from build123d import *

# Parameters (mm, degrees)
SKETCH1_R           = 6
BOSS_EXTRUDE1_DEPTH = 50
SKETCH2_R           = 5.5
CUT_EXTRUDE1_DEPTH  = 50
FILLET1_R           = 1
FILLET2_R           = 1


with BuildPart() as part:
    # Sketch1 → Boss-Extrude1 (new body)
    with BuildSketch(Plane(origin=(0, 0, 0), x_dir=(1, 0, 0), z_dir=(0, 1, 0))):
        with Locations(Location((0, 0, 0), (0, 0, 270))):
            Circle(SKETCH1_R)
    extrude(amount=BOSS_EXTRUDE1_DEPTH)

    # Sketch2 → Cut-Extrude1 (cut)
    with BuildSketch(Plane(origin=(0, 50, 0), x_dir=(1, 0, 0), z_dir=(0, 1, 0))):
        with Locations(Location((0, 0, 0), (0, 0, 270))):
            Circle(SKETCH2_R)
    extrude(amount=-CUT_EXTRUDE1_DEPTH, mode=Mode.SUBTRACT)

    # Fillet1
    # the kernel refuses this fillet: 1 mm, written as the material it takes off along each edge
    with BuildSketch(Plane(origin=(0, 50, 0), x_dir=(0, 0, 1), z_dir=(-1, 0, 0))) as fillet1_piece_1:
        with BuildLine():
            CenterArc((5, -0.866025404), FILLET1_R, 0, 60)
            Line((5.5, 0), (5.51, 0.017320508))
            ThreePointArc((5.51, 0.017320508), (5.75, 0.02), (6, 0.02))
            Line((6, 0.02), (6.02, 0))
            Line((6.02, 0), (6.02, -0.866025404))
            Line((6.02, -0.866025404), (6, -0.866025404))
        make_face()
    revolve(axis=Axis((0, 50, 0), (0, 1, 0)), mode=Mode.SUBTRACT)

    # Fillet2
    # the kernel refuses this fillet: 1 mm, written as the material it takes off along each edge
    with BuildSketch(Plane(origin=(0, 0, 0), x_dir=(0, 0, 1), z_dir=(-1, 0, 0))) as fillet2_piece_1:
        with BuildLine():
            CenterArc((5, 0.866025404), FILLET2_R, 300, 60)
            Line((5.5, 0), (5.51, -0.017320508))
            ThreePointArc((5.51, -0.017320508), (5.75, -0.02), (6, -0.02))
            Line((6, -0.02), (6.02, 0))
            Line((6.02, 0), (6.02, 0.866025404))
            Line((6.02, 0.866025404), (6, 0.866025404))
        make_face()
    revolve(axis=Axis((0, 0, 0), (0, 1, 0)), mode=Mode.SUBTRACT)


solid = part.part
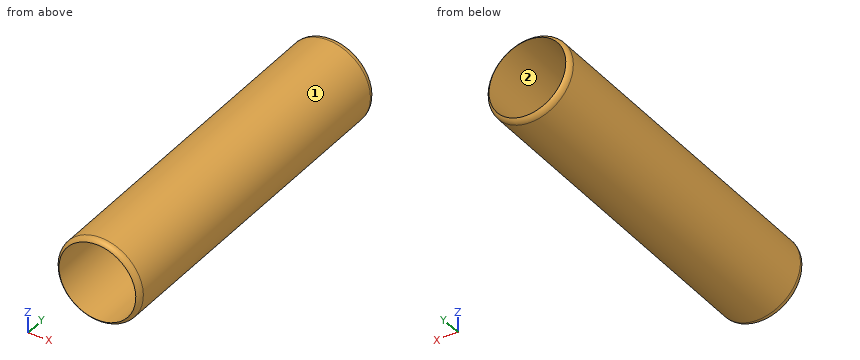
Input: part model. Units: mm. Frame: model coordinates. Face numbers are marked on the shaded views. Give positions to 0.01 mm unless a question says otherwise; leave off trailing zeros. Write each loop counter-clockwise with the first axis right and the second up, starting at its lowest first coordinate (ties: lowest second). Pieces come first, ordered by that corner, then holes. Notation, with made-up numbers: M -15.5,-23 L 32.5,-23 A7 cw 32.5,-16 Z; hole C -38,65.5 d11. An arc over 180 degrees is marked long. Use one line per item in the form item = value.
1. Ray query, L1, parallel to X at y = 10.5, z = 0; L2, parallel to Z at x = -4, y = 4; L3, parallel to X at y = 25, z = -1.5. Return the intervals inside material, ascending.
Outcome:
L1 = -6 to -5.5, 5.5 to 6
L2 = -4.47 to -3.77, 3.77 to 4.47
L3 = -5.81 to -5.29, 5.29 to 5.81
2. Cut plane C-C on y = 25. Return loops of the section in (x, z), and give its area (3 significant figures).
Outcome:
outline = C 0,0 d12; hole C 0,0 d11
area = 18.1 mm²
3. Mould query, pull axis Z, two halves, no side actions, for the marked faces 1 and 2. Classes: released by +Z, released by -Z, zero draft, split by the parting line, or undercut.
Outcome:
face_1 = split by the parting line
face_2 = undercut
4. First-contact query: P1, Ø4, axis at y = 39, z = 1, coming from the +X side; P2, Ø2, axis at x = 3.5, z = 2.5, coming from the +Y side. Flat tips, straight axial feed; report the tip coordinate or a pass-through.
Outcome:
P1 = 6
P2 = through
5. Cut plane A-A on z = 0. Return loops of the section in (x, y).
Outcome:
outline = M -6,0.87 A1 ccw -5.5,0 L -5.5,50 A1 ccw -6,49.13 Z; M 5.5,0 A1 ccw 6,0.87 L 6,49.13 A1 ccw 5.5,50 Z
6. Cut plane B-B on x = 0. Return loops of the section in (y, z).
Outcome:
outline = M 0,-5.5 A1 ccw 0.87,-6 L 49.13,-6 A1 ccw 50,-5.5 Z; M 0,5.5 L 50,5.5 A1 ccw 49.13,6 L 0.87,6 A1 ccw Z
